The listing builds one solid part. Answer for the finished solid, in the listing's coordinates (mm). A direction names the side the tool comes from. Round coordinates to 2 decimals unless told otherwise and drop trailing zeros. Loops run counter-clockwise (first coordinate to the right, second up) from the corner with the lowest first, then second, coordinate; pieces in that order, holes last. Notation, with made-up numbers: (-5, 58.25) -> (40, 58.25) arc R22 cw to (40, 78.25) -> close; hole circle Ø9 at (18.25, 41.25). An arc over 180 degrees is marked (long way). One line per question, with ' | ' between items.
from build123d import *

# Parameters (mm, degrees)
SKETCH1_W                = 10
SKETCH1_H                = 30
BOSS_EXTRUDE1_DEPTH      = 10
BOSS_EXTRUDE2_DEPTH      = 10
SKETCH4_R                = 6
BOSS_EXTRUDE3_DEPTH      = 30
BOSS_EXTRUDE4_REACH      = 57.227
BOSS_EXTRUDE4_END_RADIUS = 6
SKETCH5_R                = 4
BOSS_EXTRUDE5_REACH      = 60.949
BOSS_EXTRUDE5_END_RADIUS = 4
SKETCH7_W                = 9.610963381
SKETCH7_H                = 7.741253353
CUT_EXTRUDE1_DEPTH       = 5
CUT_EXTRUDE2_START       = -2.5
CUT_EXTRUDE2_DEPTH       = 5


# Read off the part's stored shape, not the designer's step: Cut-Extrude2
with BuildPart() as part:
    # Sketch1 → Boss-Extrude1 (new body)
    with BuildSketch(Plane(origin=(0, 0, 0), x_dir=(1, 0, 0), z_dir=(0, 1, 0))):
        Rectangle(SKETCH1_W, SKETCH1_H)
        with BuildLine():
            ThreePointArc((31.891669625, 9.819449375), (40, 0), (31.891669625, -9.819449375))
            Line((31.891669625, -9.819449375), (5, -15))
            Line((5, -15), (5, 15))
            Line((5, 15), (31.891669625, 9.819449375))
        make_face()
    extrude(amount=BOSS_EXTRUDE1_DEPTH)

    # Sketch2 → Boss-Extrude2 (add)
    with BuildSketch(Plane.ZY.offset(5)):
        with BuildLine():
            Line((-15, 10), (-9.819449375, 36.891669625))
            ThreePointArc((-9.819449375, 36.891669625), (0, 45), (9.819449375, 36.891669625))
            Line((9.819449375, 36.891669625), (15, 10))
            Line((15, 10), (-15, 10))
        make_face()
    extrude(amount=-BOSS_EXTRUDE2_DEPTH)

    # Sketch4 → Boss-Extrude3 (add)
    with BuildSketch(Plane(origin=(5, 0, 0), x_dir=(0, 0, -1), z_dir=(1, 0, 0))):
        with Locations((0, 35)):
            Circle(SKETCH4_R)
    extrude(amount=BOSS_EXTRUDE3_DEPTH)

    # Boss-Extrude4: up to this cylinder (the profile starts outside it)
    boss_extrude4_end = Plane(origin=(30, 35, 0), z_dir=(-1, 0, 0)) * Cylinder(BOSS_EXTRUDE4_END_RADIUS, 127.454, mode=Mode.PRIVATE)
    # Sketch5 → Boss-Extrude4 (add, up to the surface)
    with BuildSketch(Plane(origin=(0, 10, 0), x_dir=(1, 0, 0), z_dir=(0, 1, 0)), mode=Mode.PRIVATE) as boss_extrude4_sk1:
        with Locations(Location((30, 0, 0), (0, 0, 90))):
            Circle(SKETCH5_R)
    boss_extrude4_tool1 = extrude(boss_extrude4_sk1.sketch, amount=BOSS_EXTRUDE4_REACH, mode=Mode.PRIVATE) - boss_extrude4_end
    add(boss_extrude4_tool1.solids().sort_by_distance((30, 10, 0))[0])

    # Boss-Extrude5: up to this cylinder (the profile starts outside it)
    boss_extrude5_end = Plane(origin=(30, 20, 0), z_dir=(0, -1, 0)) * Cylinder(BOSS_EXTRUDE5_END_RADIUS, 130.898, mode=Mode.PRIVATE)
    # Sketch6 → Boss-Extrude5 (add, up to the surface)
    with BuildSketch(Plane(origin=(5, 0, 0), x_dir=(0, 0, -1), z_dir=(1, 0, 0)), mode=Mode.PRIVATE) as boss_extrude5_sk1:
        Polygon((-1.443375673, 22.5), (-2.886751346, 20), (-1.443375673, 17.5), (1.443375673, 17.5), (2.886751346, 20), (1.443375673, 22.5), align=None)
    boss_extrude5_tool1 = extrude(boss_extrude5_sk1.sketch, amount=BOSS_EXTRUDE5_REACH, mode=Mode.PRIVATE) - boss_extrude5_end
    add(boss_extrude5_tool1.solids().sort_by_distance((5, 20, 0))[0])

    # Sketch7 → Cut-Extrude1 (cut)
    with BuildSketch(Plane(origin=(5, 0, 0), x_dir=(0, 0, -1), z_dir=(1, 0, 0))):
        with Locations((0.16655936, 19.575208137)):
            Rectangle(SKETCH7_W, SKETCH7_H)
    extrude(amount=CUT_EXTRUDE1_DEPTH, mode=Mode.SUBTRACT)

    # Cut-Extrude2 outline → Cut-Extrude2 (cut)
    with BuildSketch(Plane.YZ.offset(CUT_EXTRUDE2_START)):
        with BuildLine():
            Line((43.660254038, 5), (23.660254038, 5))
            ThreePointArc((23.660254038, 5), (25, 0), (23.660254038, -5))
            Line((23.660254038, -5), (43.660254038, -5))
            ThreePointArc((43.660254038, -5), (45, 0), (43.660254038, 5))
        make_face()
    extrude(amount=CUT_EXTRUDE2_DEPTH, mode=Mode.SUBTRACT)


solid = part.part
Q1. A cutting plane is placed at C-C on y = 15. Give the vertices of the cut face in (x, z), plus the area to 3 significant figures.
Numbers:
outline: (-5, -14.04) -> (5, -14.04) -> (5, 14.04) -> (-5, 14.04) -> close; circle Ø8 at (30, 0) | area: 331 mm^2
Q2. Given pin 1 Ø9 at (y, z) = (20, 2) entering from +X; pin 2 Ø9 at (x, z) = (30.5, 7) entering from +Y; pin 3 Ø5.5 at (x, y) = (1, 36.5) entering from +Z; pin 4 Ø1.4 at (x, z) = (18, -0.5) entering from -Y, each flat-ended and moving along its own axis, determine where each tip first touches the part or whether it passes through.
Numbers:
pin 1: x = 34 | pin 2: y = 40.45 | pin 3: z = 10.42 | pin 4: y = 0
Q3. For faces 5 (the face through (33.905, 20.12, 0.867)), 6 (the face through (35, 35, 0)), 7 (the face through (18.495, 18.768, 2.175)), determine the directions among +Z, -Z, +X, -X, +Y, -Y from which every point of the face is accessible in a straight line to the end or side of a thin tool.
Numbers:
face 5: none | face 6: +Z, -Z, +X, +Y | face 7: +Z
Q4. A cutting plane is placed at B-B on x = 8. Give the vertices of the cut face in (y, z), plus the area to 3 significant figures.
Numbers:
outline: (0, -14.42) -> (10, -14.42) -> (10, 14.42) -> (0, 14.42) -> close; circle Ø12 at (35, 0) | area: 402 mm^2
Q5. A cutting plane is placed at A-A on z = 0. Give the vertices of the cut face in (x, y).
Numbers:
outline: (-5, 0) -> (40, 0) -> (40, 10) -> (34, 10) -> (34, 29) -> (35, 29) -> (35, 41) -> (5, 41) -> (5, 45) -> (2.5, 45) -> (2.5, 25) -> (-2.5, 25) -> (-2.5, 45) -> (-5, 45) -> close; hole (5, 10) -> (26, 10) -> (26, 17.5) -> (10, 17.5) -> (10, 22.5) -> (26, 22.5) -> (26, 29) -> (5, 29) -> close
Q6. A cutting plane is placed at D-D on x = 22. Give the vertices of the cut face in (y, z).
Numbers:
outline: (0, -11.73) -> (10, -11.73) -> (10, 11.73) -> (0, 11.73) -> close; (17.5, -1.44) -> (20, -2.89) -> (22.5, -1.44) -> (22.5, 1.44) -> (20, 2.89) -> (17.5, 1.44) -> close; circle Ø12 at (35, 0)
Q7. For a pull along Z with two mould halves and no side action, classify faces 1 (the face through (10, 20, 0)), 2 (the face through (0, 34, -5)), 3 (the face through (0, 25, 0)), 4 (the face through (-3, 45, 0)) as pulls with the +Z half, pulls with the -Z half, needs draft (parallel to the pull), parting line crosses it, or undercut.
Numbers:
face 1: needs draft | face 2: undercut | face 3: undercut | face 4: parting line crosses it
Q8. Find the intervals of material crossed by line 1 (Y direction, x = 25, z = -0.25); line 2 (X direction, y = 28.5, z = -4.5); line 3 (X direction, y = 18.5, z = 8), in increasing order. Write a range as from..to.
Numbers:
line 1: 0..10, 17.5..22.5, 29.01..40.99 | line 2: -5..-2.5, 2.5..5 | line 3: -5..5
